Geometry check sheet. Reference: the model listing, model coordinates, mm. A direction names the side the tool comes from. Coordinates: 2 decimals unless noted, no trailing zeros. Loops run counter-clockwise (first coordinate to the right, second up) from the corner with the lowest first, then second, coordinate; pieces in that order, holes last.
from build123d import *

# Parameters (mm, degrees)
SKETCH_1_W          = 118.3
SKETCH_1_H          = 31.5
EXTRUDE_1_DEPTH     = 2.8
CUT_EXTRUDE_1_DEPTH = 122.787422537
SKETCH_3_W          = 2.8
SKETCH_3_H          = 31.5
CUT_EXTRUDE_2_DEPTH = 1


with BuildPart() as part:
    # 草图1 → 凸台-拉伸1 (new body)
    with BuildSketch(Plane(origin=(0, 0, 0), x_dir=(1, 0, 0), z_dir=(0, 1, 0))):
        with Locations((4.649344978, 13.05010917)):
            Rectangle(SKETCH_1_W, SKETCH_1_H)
    extrude(amount=EXTRUDE_1_DEPTH)

    # 草图2 → 切除-拉伸1 (cut, through all)
    with BuildSketch(Plane(origin=(63.799344978, 0, 0), x_dir=(0, 0, -1), z_dir=(1, 0, 0))):
        Polygon((-2.69989083, 0), (-2.69989083, 2.8), (0.10010917, 2.8), align=None)
    extrude(amount=-CUT_EXTRUDE_1_DEPTH, mode=Mode.SUBTRACT)

    # 草图3 → 切除-拉伸2 (cut)
    with BuildSketch(Plane(origin=(0, 2.8, 0), x_dir=(1, 0, 0), z_dir=(0, 1, 0))):
        with Locations((-53.100655022, 13.05010917)):
            Rectangle(SKETCH_3_W, SKETCH_3_H)
        with Locations((62.399344978, 13.05010917)):
            Rectangle(SKETCH_3_W, SKETCH_3_H)
    extrude(amount=-CUT_EXTRUDE_2_DEPTH, mode=Mode.SUBTRACT)


solid = part.part
1) Depth check by flat-ended pin: pin 1 (0.5 mm diameter, centred on y = 2.5, z = -9.5, fed in from +X); pin 2 (0.8 mm diameter, centred on x = -53.5, z = -21, fed in from +Y). Enter the tip coordinate at first touch or a pass-through.
Data:
pin 1: stops at x = 61
pin 2: stops at y = 1.8
2) Access from +Z, -Z, +X, -X, +Y, -Y to the whole of each face (thin tool, end or side, straight path). Record for faces 1 (the flat face through (4, 2.8, -15)), 2 (the flat face through (-53, 1.8, -14)), 3 (the flat face through (62, 1.8, -14)).
Data:
face 1: +Z, -Z, +X, -X, +Y
face 2: +Z, -Z, -X, +Y
face 3: +Z, -Z, +X, +Y
3) Section check C-C on y = 0.8. Record the cut outline in (x, z).
Data:
outline: (-54.5, -28.8) - (63.8, -28.8) - (63.8, 1.9) - (-54.5, 1.9) - close
4) Material ranges on probe 1 along X at (y, z) = (2.1, -7); probe 2 along Z at (x, y) = (13.5, 0.15); probe 3 along Z at (x, y) = (32.5, 2.15), recorded low to high.
Data:
probe 1: x = -51.7 to 61
probe 2: z = -28.8 to 2.55
probe 3: z = -28.8 to 0.55
5) Section check B-B on x = -4. Record the cut outline in (y, z), and give its area (3 significant figures).
Data:
outline: (0, -28.8) - (2.8, -28.8) - (2.8, -0.1) - (0, 2.7) - close
area: 84.3 mm2
6) Section check A-A on z = -10.5. Record the cut outline in (x, y), and give its area (3 significant figures).
Data:
outline: (-54.5, 0) - (63.8, 0) - (63.8, 1.8) - (61, 1.8) - (61, 2.8) - (-51.7, 2.8) - (-51.7, 1.8) - (-54.5, 1.8) - close
area: 326 mm2
